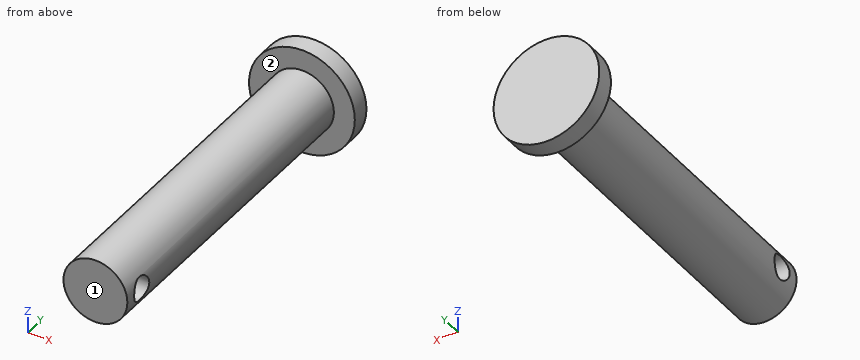
```python
from build123d import *

# Parameters (mm, degrees)
SKETCH1_R               = 2.9
BOSS_EXTRUDE1_DEPTH     = 30.15
SKETCH2_R               = 4.8
BOSS_EXTRUDE2_DEPTH     = 1.7
SKETCH3_R               = 1.1
CUT_EXTRUDE1_DEPTH      = 5.8
CUT_EXTRUDE1_DEPTH_BACK = 5.8


with BuildPart() as part:
    # Sketch1 → Boss-Extrude1 (new body)
    with BuildSketch(Plane(origin=(0, 0, 0), x_dir=(1, 0, 0), z_dir=(0, 1, 0))):
        Circle(SKETCH1_R)
    extrude(amount=-BOSS_EXTRUDE1_DEPTH)

    # Sketch2 → Boss-Extrude2 (add)
    with BuildSketch(Plane(origin=(0, 0, 0), x_dir=(1, 0, 0), z_dir=(0, 1, 0))):
        Circle(SKETCH2_R)
    extrude(amount=BOSS_EXTRUDE2_DEPTH)

    # Sketch3 → Cut-Extrude1 (cut, two sides)
    with BuildSketch(Plane(origin=(0, 0, 0), x_dir=(0, 0, -1), z_dir=(1, 0, 0))) as cut_extrude1_sk:
        with Locations((0, -28.05)):
            Circle(SKETCH3_R)
    extrude(amount=CUT_EXTRUDE1_DEPTH, mode=Mode.SUBTRACT)
    extrude(cut_extrude1_sk.sketch, amount=-CUT_EXTRUDE1_DEPTH_BACK, mode=Mode.SUBTRACT)


solid = part.part
```
Geometry check sheet. Reference: the model listing, model coordinates, mm. Face numbers are marked on the shaded views. A direction names the side the tool comes from. Coordinates: 2 decimals unless noted, no trailing zeros. Order: outer loops, then holes, each group sorted by start corner. A loop starts at its lowest first (then second) coordinate and runs counter-clockwise, first axis right, second up. Notation, with made-up numbers: M 32,-27 L 56,-27 A22 ccw 56,9 Z; hole C 87,-26 d1. An arc over 180 degrees is marked long. One line per question, with ' | ' between items. Start each with the question number.
Item 1: Material ranges on L1, parallel to Y at x = -1.75, z = 0; L2, parallel to Z at x = -1.4, y = -28.05; L3, parallel to Y at x = -3.5, z = 1.5, recorded low to high. Write a range as [from, to].
Item 2: Cross-section at B-B on y = -28.05. Enter the section's corners in (x, z), then the cut area to 3 significant figures.
Item 3: Set-up check for the marked faces 1 and 2: record each of +Z, -Z, +X, -X, +Y, -Y from which the full face is reachable in a straight line by a thin tool's end or side.
Item 4: Cross-section at A-A on x = 2. Enter the section's corners in (y, z), then the cut area to 3 significant figures.
Item 5: Cross-section at C-C on x = -1.5. Enter the section's corners in (y, z), then the cut area to 3 significant figures.
Item 6: Gauge pin test, flat ends, axial feed: pin 1 (1 mm diameter, centred on y = -20.5, z = -0.5, fed in from +X); pin 2 (1 mm diameter, centred on y = -2.5, z = -1.5, fed in from -X); pin 3 (1.3 mm diameter, centred on y = -28.05, z = 0, fed in from +X); pin 4 (1 mm diameter, centred on x = -3, y = -26.5, fed in from +Z). Record the tip position at first contact, or that the pin passes through.
Item 7: Cross-section at D-D on z = 4. Enter the section's corners in (x, y).
Findings:
1) L1: y = [-30.15, -29.15], [-26.95, 1.7] | L2: z = [-2.54, -1.1], [1.1, 2.54] | L3: y = [0, 1.7]
2) outline: M -2.68,-1.1 A2.9 ccw 2.68,-1.1 Z; M -2.68,1.1 L 2.68,1.1 A2.9 ccw Z | area: 14.0 mm²
3) face 1: +Z, -Z, +X, -X, -Y | face 2: -Y
4) outline: M -30.15,-2.1 L 0,-2.1 L 0,-4.36 L 1.7,-4.36 L 1.7,4.36 L 0,4.36 L 0,2.1 L -30.15,2.1 Z; hole C -28.05,0 d2.2 | area: 138 mm²
5) outline: M -30.15,-2.48 L 0,-2.48 L 0,-4.56 L 1.7,-4.56 L 1.7,4.56 L 0,4.56 L 0,2.48 L -30.15,2.48 Z; hole C -28.05,0 d2.2 | area: 161 mm²
6) pin 1: stops at x = 2.9 | pin 2: stops at x = -2.72 | pin 3: passes through | pin 4: stops at z = 1.47
7) outline: M -2.65,0 L 2.65,0 L 2.65,1.7 L -2.65,1.7 Z
